Autodesk Inventor part; units mm, degrees
ref_plane "YZ Plane" through (0, 0, 0) normal (1, 0, 0) x (0, 1, 0)
ref_plane "XZ Plane" through (0, 0, 0) normal (0, 1, 0) x (-1, 0, 0)
ref_plane "XY Plane" through (0, 0, 0) normal (0, 0, 1) x (1, 0, 0)
sketch "スケッチ1" plane through (0, 0, 0) normal (0, 0, 1) x (1, 0, 0)
  circle A0 centre (0, 0) radius 1.9
  dimension "d0" = 3.8
extrude "押し出し1" add sketch "スケッチ1" along normal blind 1.3
sketch "スケッチ2" plane through (0, 0, 0) normal (0, 0, -1) x (-1, 0, 0)
  circle A0 centre (0, 0) radius 1.9
  circle A1 centre (0, 0) radius 1
  dimension "d3" = 2
extrude "押し出し2" add sketch "スケッチ2" along normal blind 6 contours A1
sketch "スケッチ3" plane through (0, 0, 1.3) normal (0, 0, 1) x (1, 0, 0)
  circle A0 centre (0, 0) radius 1.9
  line L0 (0, 0.866) -> (0.75, 0.433)
  line L1 (0.75, 0.433) -> (0.75, -0.433)
  line L2 (0.75, -0.433) -> (0, -0.866)
  line L3 (0, -0.866) -> (-0.75, -0.433)
  line L4 (-0.75, -0.433) -> (-0.75, 0.433)
  line L5 (-0.75, 0.433) -> (0, 0.866)
  dimension "d6" = 0.75
extrude "押し出し3" cut sketch "スケッチ3" against normal blind 1.5 contours L0 L1 L2 L3 L4 L5
fillet "フィレット1" radius 0.3 2 edges at (-1.9, 0, 1.3) (-1.9, 0, 0)
fillet "フィレット2" radius 0.1 19 edges at (-0.375, 0.6495, 1.3) (-0.75, 0, 1.3) (-0.375, -0.6495, 1.3) (0.375, -0.6495, 1.3) (0.75, 0, 1.3) (0.375, 0.6495, 1.3) (-0.375, 0.6495, -0.2) (0.375, 0.6495, -0.2) (0, 0.866, 0.55) (-0.75, 0.433, 0.55) (-0.375, -0.6495, -0.2) (-0.75, -0.433, 0.55) (-0.75, 0, -0.2) (0.75, 0, -0.2) (0.75, 0.433, 0.55) (0.75, -0.433, 0.55) (0.375, -0.6495, -0.2) (0, -0.866, 0.55) (1, 0, -6)
thread "ねじ3"
Geometry: final body of the model. Coordinates: model frame, mm. A direction names the side the tool comes from. Coordinates: 2 decimals unless noted, no trailing zeros. Loops run counter-clockwise (first coordinate to the right, second up) from the corner with the lowest first, then second, coordinate; pieces in that order, holes last. Notation, with made-up numbers: (6, -17.5) - (26, -17.5) arc R35 cw to (26, 19.5) - close; hole circle Ø6 at (-25, 79.5). An arc over 180 degrees is marked (long way). One line per question, with ' | ' between items. Start each with the question number.
(1) Reachability of faces 1 (the flat face through (-1, -1, 0)), 2 (the flat face through (0, 0, -6)) from +Z, -Z, +X, -X, +Y, -Y: full face, straight path, thin tool, end or side. Return the list, or none.
(2) Ray query, L1, parallel to Z at x = 0.25, y = -0.55; L2, parallel to Y at x = -1.7, z = 1; L3, parallel to Y at x = -0.7, z = 1. Return the intervals inside material, ascending. Write a range as from..to.
(3) Cut plane A-A on y = 0. Output: boundary loops of the cut face in (x, z), and give its area (3 significant figures).
(4) First-contact query: pin 1 (1 mm diameter, centred on y = -0.5, z = -1, fed in from +X); pin 2 (1 mm diameter, centred on x = 1, z = -3.5, fed in from -Y); pin 3 (2 mm diameter, centred on x = -0.5, z = -4.5, fed in from -Y). Flat tips, straight axial feed; report the tip coordinate or a pass-through.
(5) Draft query along Y for faces 3 (the flat face through (1, -1, 1.3)), 4 (the cylindrical face through (-1.9, -0.08, 0.65)), 5 (the flat face through (0, 0, -0.2)). Return one class per face: +Y half, -Y half, draft (parallel to the pull), parting line (faces both ways), or undercut.
(6) Cut plane B-B on z = -4.75. Output: boundary loops of the cut face in (x, y).
Here are the results:
1) face 1: -Z | face 2: -Z, +X, -X, +Y, -Y
2) L1: -6..-0.2 | L2: -0.85..0.85 | L3: -1.77..-0.46, 0.46..1.77
3) outline: (-1.9, 0.3) arc R0.3 ccw to (-1.6, 0) - (-1, 0) - (-1, -5.9) arc R0.1 ccw to (-0.9, -6) - (0.9, -6) arc R0.1 ccw to (1, -5.9) - (1, 0) - (1.6, 0) arc R0.3 ccw to (1.9, 0.3) - (1.9, 1) arc R0.3 ccw to (1.6, 1.3) - (0.85, 1.3) arc R0.1 ccw to (0.75, 1.2) - (0.75, -0.1) arc R0.1 cw to (0.65, -0.2) - (-0.65, -0.2) arc R0.1 cw to (-0.75, -0.1) - (-0.75, 1.2) arc R0.1 ccw to (-0.85, 1.3) - (-1.6, 1.3) arc R0.3 ccw to (-1.9, 1) - close | area: 14.6 mm²
4) pin 1: x = 1 | pin 2: y = -0.87 | pin 3: y = -1
5) face 3: draft | face 4: parting line | face 5: undercut
6) outline: circle Ø2 at (0, 0)
